Build history of the part. All positions in model axes, mm. A direction names the side the tool comes from. Give positions to 0.01 mm unless a question says otherwise; leave off trailing zeros. Write each loop counter-clockwise with the first axis right and the second up, starting at its lowest first coordinate (ties: lowest second). Pieces come first, ordered by that corner, then holes. Notation, with made-up numbers: (44.25, 18.25) -> (74.25, 18.25) arc R24 ccw to (74.25, 41.25) -> close; hole circle Ø5 at (-16.5, -29.75). An arc over 180 degrees is marked (long way). Put each result on its own line as item: value. Start each with the question number.
Item 1: Slice it at B-B, the plane z = 0. List the corners of the cut face in (x, y).
Item 2: Slice it at C-C, the plane y = 1.5. List the corners of the cut face in (x, z).
Item 3: Drill centre lines: line 1 along Z through (x, y) = (-35.25, 1.6); line 2 along Z through (x, y) = (35.25, 0.9); line 3 along X through (y, z) = (0.1, 0.5). Where is each one in solid material? Low to high.
Item 4: Slice it at D-D, the plane x = 35.25. List the corners of the cut face in (y, z).
Item 5: Tool access for faces 1 (the flat face through (11, 2.5, 0)), 2 (the cylindrical face through (-32.88, 1.23, -2.1)), 3 (the cylindrical face through (-32.858, 1.232, 2.094)): list every direction of +Z, -Z, +X, -X, +Y, -Y with a clear straight run to the whole face (end or side of a thin tool).
Item 6: Two-plate mould, pull along Z, no slides. Class faces 4 (the cylindrical face through (34.06, 1.27, 0.91)), 5 (the cylindrical face through (41.746, 1.232, -0.224)), 6 (the cylindrical face through (29.21, 1.23, 3.31)): pulls with the +Z half, pulls with the -Z half, needs draft (parallel to the pull), parting line crosses it, or undercut.
Item 7: Flat gauge pins, fed straight in: pin 1 Ø1.5 at (x, y) = (21, 1.5) entering from -Z; pin 2 Ø4 at (x, z) = (-19.5, 5) entering from +Y; pin 3 Ø1 at (x, y) = (-24.5, 1) entering from +Z; pin 4 Ø1 at (x, y) = (4.5, 2) entering from -Z. Where does each tip first touch, or does it go through?
Item 8: Slice it at A-A, the plane x = -35.25. List the corners of the cut face in (y, z), plus the area to 4 significant figures.
```python
from build123d import *

# Parameters (mm, degrees)
BOSS_EXTRUDE1_DEPTH = 2.5
CUT_EXTRUDE1_REACH  = 4.5
SKETCH2_R           = 0.75
SKETCH2_R_2         = 1.5


with BuildPart() as part:
    # Sketch1 → Boss-Extrude1 (new body)
    with BuildSketch(Plane(origin=(0, 0, 0), x_dir=(1, 0, 0), z_dir=(0, 1, 0))):
        with BuildLine():
            Line((-32.216386231, 2), (27.934070474, 3))
            ThreePointArc((27.934070474, 3), (29.194347957, 3.300786008), (30.210243769, 4.104979553))
            ThreePointArc((30.210243769, 4.104979553), (41.75, 0), (30.210243769, -4.104979553))
            ThreePointArc((30.210243769, -4.104979553), (29.194347957, -3.300786008), (27.934070474, -3))
            Line((27.934070474, -3), (-32.216386231, -2))
            ThreePointArc((-32.216386231, -2), (-32.86638269, -2.097194277), (-33.449778955, -2.3998342))
            ThreePointArc((-33.449778955, -2.3998342), (-38.25, 0), (-33.449778955, 2.3998342))
            ThreePointArc((-33.449778955, 2.3998342), (-32.86638269, 2.097194277), (-32.216386231, 2))
        make_face()
    extrude(amount=BOSS_EXTRUDE1_DEPTH)

    # Sketch2 → Cut-Extrude1 (cut, up to next)
    with BuildSketch(Plane(origin=(0, 2.5, 0), x_dir=(1, 0, 0), z_dir=(0, 1, 0)), mode=Mode.PRIVATE) as cut_extrude1_sk1:
        with Locations((-35.25, 0)):
            Circle(SKETCH2_R)
    cut_extrude1_tool1 = extrude(cut_extrude1_sk1.sketch, amount=-CUT_EXTRUDE1_REACH, mode=Mode.PRIVATE) & part.part
    add(cut_extrude1_tool1.solids().sort_by_distance((-35.25, 2.5, 0))[0], mode=Mode.SUBTRACT)
    # Sketch2 → Cut-Extrude1 (cut, up to next)
    with BuildSketch(Plane(origin=(0, 2.5, 0), x_dir=(1, 0, 0), z_dir=(0, 1, 0)), mode=Mode.PRIVATE) as cut_extrude1_sk2:
        with Locations((35.25, 0)):
            Circle(SKETCH2_R_2)
    cut_extrude1_tool2 = extrude(cut_extrude1_sk2.sketch, amount=-CUT_EXTRUDE1_REACH, mode=Mode.PRIVATE) & part.part
    add(cut_extrude1_tool2.solids().sort_by_distance((35.25, 2.5, 0))[0], mode=Mode.SUBTRACT)


solid = part.part
```
Values follow:
1. outline: (-38.25, 0) -> (-36, 0) -> (-36, 2.5) -> (-38.25, 2.5) -> close; (-34.5, 0) -> (33.75, 0) -> (33.75, 2.5) -> (-34.5, 2.5) -> close; (36.75, 0) -> (41.75, 0) -> (41.75, 2.5) -> (36.75, 2.5) -> close
2. outline: (-33.45, -2.4) arc R2 cw to (-32.22, -2) -> (27.93, -3) arc R3 cw to (30.21, -4.1) arc R6.5 ccw (long way) to (30.21, 4.1) arc R3 cw to (27.93, 3) -> (-32.22, 2) arc R2 cw to (-33.45, 2.4) arc R3 ccw (long way) to start; hole circle Ø1.5 at (-35.25, 0); hole circle Ø3 at (35.25, 0)
3. line 1: -3 to -0.75, 0.75 to 3
3. line 2: -6.5 to -1.5, 1.5 to 6.5
3. line 3: -38.21 to -35.81, -34.69 to 33.84, 36.66 to 41.73
4. outline: (0, -6.5) -> (2.5, -6.5) -> (2.5, -1.5) -> (0, -1.5) -> close; (0, 1.5) -> (2.5, 1.5) -> (2.5, 6.5) -> (0, 6.5) -> close
5. face 1: +Z, -Z, +X, -X, +Y
5. face 2: -Z, +Y, -Y
5. face 3: +Z, +Y, -Y
6. face 4: undercut
6. face 5: parting line crosses it
6. face 6: pulls with the +Z half
7. pin 1: z = -2.9
7. pin 2: through
7. pin 3: z = 2.14
7. pin 4: z = -2.62
8. outline: (0, -3) -> (2.5, -3) -> (2.5, -0.75) -> (0, -0.75) -> close; (0, 0.75) -> (2.5, 0.75) -> (2.5, 3) -> (0, 3) -> close
8. area: 11.25 mm2
